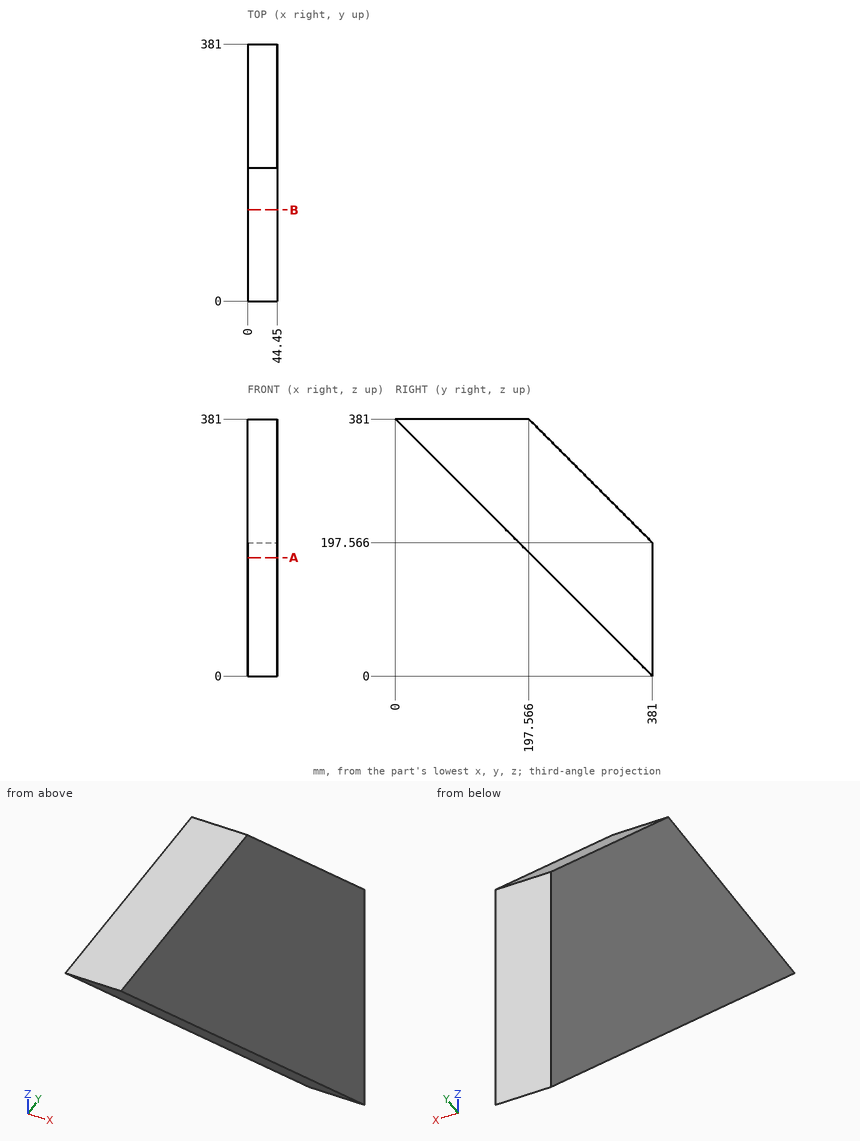
Geometry check sheet. Reference: drawing and pictorial views, mm from the part's lowest x, y, z. Coordinates: 2 decimals unless noted, no trailing zeros. Loops run counter-clockwise (first coordinate to the right, second up) from the corner with the lowest first, then second, coordinate; pieces in that order, holes last. Notation, with made-up numbers: (28, 23) -> (81, 23) arc R23 cw to (81, 32) -> close; hole circle Ø5 at (-20.75, 55.25). An arc over 180 degrees is marked (long way). Write item = value, one per line. Start each with the question number.
1. Section check B-B on y = 135. Record the cut outline in (x, z).
2. Section check A-A on z = 175.5. Record the cut outline in (x, y), then the cut area to 3 significant figures.
3. Material ranges on line 1 (Z direction, x = 8, y = 46.5); line 2 (Z direction, x = 22.5, y = 352.5) (1 decimal); line 3 (Y direction, x = 22, z = 108), recorded low to high.
4. Depth check by flat-ended pin: P1, Ø10, axis at x = 18, y = 143.5, coming from the -Z side; P2, Ø1, axis at x = 35.5, z = 273.5, coming from the +Y side (1 decimal); P3, Ø10, axis at x = 13, z = 264.5, coming from the -Y side. Enter the tip coordinate at first touch or a pass-through.
Responses:
q1.outline = (0, 246) -> (44.45, 246) -> (44.45, 381) -> (0, 381) -> close
q2.outline = (0, 205.5) -> (44.45, 205.5) -> (44.45, 381) -> (0, 381) -> close
q2.area = 7,800 mm2
q3.line_1 = 334.5 to 381
q3.line_2 = 28.5 to 226.1
q3.line_3 = 273 to 381
q4.P1 = 232.5
q4.P2 = 305.6
q4.P3 = 111.5
